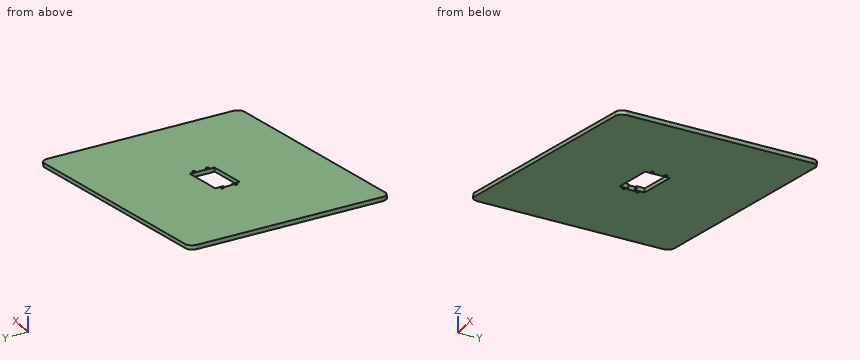
```python
from build123d import *

# Parameters (mm, degrees)
SKETCH1_W           = 355.39931416
SKETCH1_H           = 250
BOSS_EXTRUDE1_DEPTH = 5
CUT_EXTRUDE1_DEPTH  = 10
SKETCH3_R           = 2
CUT_EXTRUDE2_DEPTH  = 5
FILLET1_R           = 10


with BuildPart() as part:
    # Sketch1 → Boss-Extrude1 (new body)
    with BuildSketch(Plane(origin=(-21.339939358, 0, -121.024810115), x_dir=(-0.984807753, 0, 0.173648178), z_dir=(-0.173648178, 0, -0.984807753))):
        with Locations((-4.932202266, -11.228757924)):
            Rectangle(SKETCH1_W, SKETCH1_H)
    extrude(amount=BOSS_EXTRUDE1_DEPTH)

    # Sketch2 → Cut-Extrude1 (cut)
    with BuildSketch(Plane(origin=(-21.339939358, 0, -121.024810115), x_dir=(0.984807753, 0, -0.173648178), z_dir=(0.173648178, 0, 0.984807753))):
        Polygon((-25.067797734, -16.228757924), (-25.067797734, -26.578757924), (34.932202266, -26.578757924), (34.932202266, 4.121242076), (-25.067797734, 4.121242076), (-25.067797734, -6.228757924), (-28.067797734, -6.228757924), (-28.067797734, -16.228757924), align=None)
    extrude(amount=-CUT_EXTRUDE1_DEPTH, mode=Mode.SUBTRACT)

    # Sketch3 → Cut-Extrude2 (cut)
    with BuildSketch(Plane(origin=(-22.208180247, 0, -125.94884888), x_dir=(-0.984807753, 0, 0.173648178), z_dir=(-0.173648178, 0, -0.984807753))):
        with Locations((28.567797734, -19.678757924)):
            Circle(SKETCH3_R)
        with Locations((28.567797734, -2.778757924)):
            Circle(SKETCH3_R)
        with Locations((-38.432202266, -2.778757924)):
            Circle(SKETCH3_R)
        with Locations((-38.432202266, -19.678757924)):
            Circle(SKETCH3_R)
    extrude(amount=-CUT_EXTRUDE2_DEPTH, mode=Mode.SUBTRACT)

    # Fillet1
    fillet1_edges = [part.edges().sort_by_distance(p)[0] for p in [
        (158.083211229, 113.771242076, -155.200519056),
        (-191.916788771, 113.771242076, -93.486075809),
        (-191.916788771, -136.228757924, -93.486075809),
        (158.083211229, -136.228757924, -155.200519056),
    ]]
    fillet(fillet1_edges, radius=FILLET1_R)


solid = part.part
```
The model under review builds one solid part; all positions refer to its coordinate system, in mm. Give positions to 0.01 mm unless a question says otherwise; leave off trailing zeros. Write each loop counter-clockwise with the first axis right and the second up, starting at its lowest first coordinate (ties: lowest second). Pieces come first, ordered by that corner, then holes. Notation, with made-up numbers: (-29.75, 42) -> (-13.75, 42) arc R25 cw to (-13.75, 69) -> close; hole circle Ø6 at (20, 27). An arc over 180 degrees is marked (long way). Put each result on its own line as item: value.
(1) We need section A-A, the plane y = 65. Give the boundary of the cut face in (x, z).
Results are:
outline: (-192.35, -95.95) -> (157.65, -157.66) -> (158.52, -152.74) -> (-191.48, -91.02) -> close
(2) We need section B-B, the plane z = -138.5. Give the boundary of the cut face in (x, y), and give its area (3 significant figures).
Results are:
outline: (48.97, -136.23) -> (77.77, -136.23) -> (77.77, 113.77) -> (48.97, 113.77) -> close
area: 7,200 mm²
(3) To check wall thickness, follow probe 1 along Z at (x, y) = (52, 5); probe 2 along Z at (x, y) = (-35, -78). State the ranges of each line that lie inside material, in increasing order. Write a range as from..to.
Results are:
probe 1: -139.03..-133.96
probe 2: -123.69..-118.62
(4) For pin 1 Ø6 at (x, y) = (-152, -94.5) entering from -Z; pin 2 Ø1.5 at (x, y) = (103, 40) entering from +Z; pin 3 Ø1 at (x, y) = (-94, -58) entering from -Z, all flat-tipped, find the tip position at first contact; note any pin that passes through.
Results are:
pin 1: z = -103.59
pin 2: z = -142.82
pin 3: z = -113.38
